from build123d import *

# Parameters (mm, degrees)
SKETCH_1_W          = 35
SKETCH_1_H          = 39
SKETCH_1_R          = 2
EXTRUDE_1_DEPTH     = 8
SKETCH_2_R          = 1.65
CUT_EXTRUDE_1_DEPTH = 54.009433123


with BuildPart() as part:
    # 草图1 → 凸台-拉伸1 (new body)
    with BuildSketch(Plane.XY):
        with Locations((17.5, 19.5)):
            Rectangle(SKETCH_1_W, SKETCH_1_H)
        with Locations((17.5, 23.5)):
            Circle(SKETCH_1_R, mode=Mode.SUBTRACT)
    extrude(amount=EXTRUDE_1_DEPTH)

    # 草图2 → 切除-拉伸1 (cut, through all)
    with BuildSketch(Plane(origin=(0, 39, 0), x_dir=(1, 0, 0), z_dir=(0, 1, 0))):
        with Locations(Location((5, -4, 0), (0, 0, 270))):
            Circle(SKETCH_2_R)
        with Locations(Location((30, -4, 0), (0, 0, 270))):
            Circle(SKETCH_2_R)
    extrude(amount=-CUT_EXTRUDE_1_DEPTH, mode=Mode.SUBTRACT)


solid = part.part
Verification items for the finished model (mm, model axes). Coordinates: 2 decimals unless noted, no trailing zeros. Loops run counter-clockwise (first coordinate to the right, second up) from the corner with the lowest first, then second, coordinate; pieces in that order, holes last. Notation, with made-up numbers: (52.25, 84.25) -> (78.25, 84.25) arc R8 cw to (78.25, 90.25) -> close; hole circle Ø5 at (58, -40). An arc over 180 degrees is marked (long way). Answer as a JSON object with one key per item and string values. Group by question number.
Item 1: Sectioned sample at C-C on x = 30. Record the boundary of the cut face in (y, z).
Item 2: Mould release check, pull along X, two halves, no side actions. Record for faces 1 (the flat face through (0, 19, 4)), 2 (the flat face through (17, 20, 0)), 3 (the cylindrical face through (31.636, 19.773, 3.785)), 4 (the cylindrical face through (3.4, 19.8, 3.6)): +X half, -X half, draft (parallel to the pull), parting line (faces both ways), or undercut.
Item 3: Sectioned sample at A-A on z = 4. Record the boundary of the cut face in (x, y), plus the area to 3 significant figures.
Item 4: Sectioned sample at B-B on y = 23.5. Record the boundary of the cut face in (x, z).
Item 5: Scan lines: probe 1 along X at (y, z) = (10, 4); probe 2 along Y at (x, z) = (17.5, 2.25); probe 3 along X at (y, z) = (25, 4). Record each from-to range of solid material in increasing order.
Item 6: Sectioned sample at D-D on y = 4.5. Record the boundary of the cut face in (x, z).
Evaluation:
{
 "1": {"outline": "(0, 0) -> (39, 0) -> (39, 2.35) -> (0, 2.35) -> close; (0, 5.65) -> (39, 5.65) -> (39, 8) -> (0, 8) -> close"},
 "2": {"face 1": "-X half", "face 2": "draft", "face 3": "undercut", "face 4": "undercut"},
 "3": {"outline": "(0, 0) -> (3.35, 0) -> (3.35, 39) -> (0, 39) -> close; (6.65, 0) -> (28.35, 0) -> (28.35, 39) -> (6.65, 39) -> close; (31.65, 0) -> (35, 0) -> (35, 39) -> (31.65, 39) -> close; hole circle Ø4 at (17.5, 23.5)", "area": "1,100 mm²"},
 "4": {"outline": "(0, 0) -> (15.5, 0) -> (15.5, 8) -> (0, 8) -> close; (19.5, 0) -> (35, 0) -> (35, 8) -> (19.5, 8) -> close; hole circle Ø3.3 at (5, 4); hole circle Ø3.3 at (30, 4)"},
 "5": {"probe 1": "x = 0 to 3.35, 6.65 to 28.35, 31.65 to 35", "probe 2": "y = 0 to 21.5, 25.5 to 39", "probe 3": "x = 0 to 3.35, 6.65 to 16.18, 18.82 to 28.35, 31.65 to 35"},
 "6": {"outline": "(0, 0) -> (35, 0) -> (35, 8) -> (0, 8) -> close; hole circle Ø3.3 at (5, 4); hole circle Ø3.3 at (30, 4)"}
}
